from build123d import *

# Parameters (mm, degrees)
F0_R     = 50.5
F0_R_2   = 45.5
F1_DEPTH = 6
F2_DEPTH = 3
F3_R     = 18
F4_DEPTH = 6.001
F5_SIZE  = 1


with BuildPart() as f1:
    # F0 (on Top) → F1 (new body)
    with BuildSketch(Plane.XY):
        Circle(F0_R)
        Circle(F0_R_2, mode=Mode.SUBTRACT)
        Circle(F0_R_2)
    extrude(amount=F1_DEPTH)

    # F0 (on Top) → F2 (cut)
    with BuildSketch(Plane.XY):
        Circle(F0_R_2)
    extrude(amount=F2_DEPTH, mode=Mode.SUBTRACT)

    # F3 (on face) → F4 (cut, through all)
    with BuildSketch(Plane.XY.offset(6)):
        Circle(F3_R)
    extrude(amount=-F4_DEPTH, mode=Mode.SUBTRACT)

    # F5
    f5_edges = [f1.edges().sort_by_distance(p)[0] for p in [
        (-18, 0, 6),
        (-50.5, 0, 6),
    ]]
    chamfer(f5_edges, length=F5_SIZE)


solid = f1.part
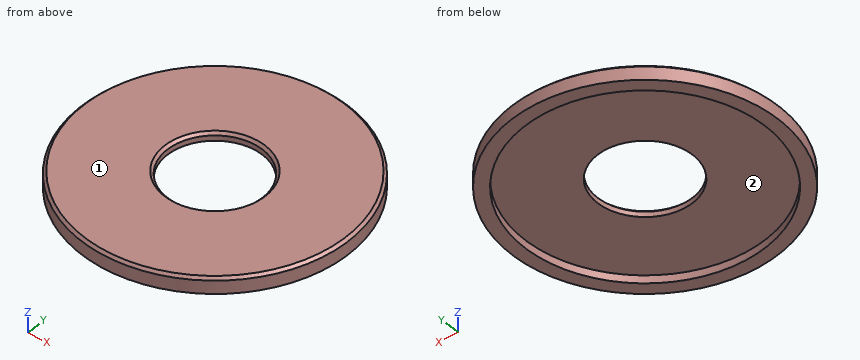
Here's how the part is built. I have some questions about the finished solid (model axes, mm). Face numbers are marked on the shaded views. Give positions to 0.01 mm unless a question says otherwise; leave off trailing zeros. Loops run counter-clockwise (first coordinate to the right, second up) from the corner with the lowest first, then second, coordinate; pieces in that order, holes last. Notation, with made-up numbers: (81.25, -33.5) -> (127.25, -33.5) arc R27 ccw to (127.25, -15.5) -> close; hole circle Ø10 at (68.5, 85.5). An arc over 180 degrees is marked (long way). Answer as a JSON object with one key per item and string values. Group by question number.
Item 1: I need wall thicknesses on L1, parallel to Y at x = 0, z = 3.4; L2, parallel to Y at x = 0, z = 2.15; L3, parallel to Z at x = -37.5, y = -10.5. Which ranges of each line are inside material? Lowest first, please.
Item 2: Thinking about a two-plate mould opening in X: for the marked faces 1 and 2, which applies, pulls with the +X half, pulls with the -X half, needs draft (parallel to the pull), parting line crosses it, or undercut?
Item 3: Will this pin go through, and if not, where does the flat tip stop? pin 1 (8 mm diameter, centred on x = 34.5, y = -5.5, fed in from -Z).
Item 4: Imagine slicing it at A-A on x = 0. Write out the boundary of the cut face in (y, z), then the cut area to 3 significant figures.
Answer list:
{
 "1": {"L1": "y = -50.5 to -18, 18 to 50.5", "L2": "y = -50.5 to -45.5, 45.5 to 50.5", "L3": "z = 3 to 6"},
 "2": {"face 1": "needs draft", "face 2": "undercut"},
 "3": {"pin 1": "stops at z = 3"},
 "4": {"outline": "(-50.5, 0) -> (-45.5, 0) -> (-45.5, 3) -> (-18, 3) -> (-18, 5) -> (-19, 6) -> (-49.5, 6) -> (-50.5, 5) -> close; (18, 3) -> (45.5, 3) -> (45.5, 0) -> (50.5, 0) -> (50.5, 5) -> (49.5, 6) -> (19, 6) -> (18, 5) -> close", "area": "223 mm2"}
}
